```python
from build123d import *

# Parameters (mm, degrees)
SKETCH1_R           = 131
SKETCH1_R_2         = 126
BOSS_EXTRUDE1_DEPTH = 280
SKETCH4_R           = 140
SKETCH4_R_2         = 131
BOSS_EXTRUDE2_DEPTH = 9
CHAMFER1_SIZE       = 20
CHAMFER1_SIZE2      = 3.526539614
SKETCH5_R           = 132
SKETCH5_R_2         = 131
BOSS_EXTRUDE3_DEPTH = 15


with BuildPart() as part:
    # Sketch1 → Boss-Extrude1 (new body)
    with BuildSketch(Plane(origin=(0, 0, 0), x_dir=(1, 0, 0), z_dir=(0, 1, 0))):
        Circle(SKETCH1_R)
        Circle(SKETCH1_R_2, mode=Mode.SUBTRACT)
    extrude(amount=-BOSS_EXTRUDE1_DEPTH)

    # Sketch4 → Boss-Extrude2 (add)
    with BuildSketch(Plane(origin=(0, -12, 0), x_dir=(1, 0, 0), z_dir=(0, 1, 0))):
        Circle(SKETCH4_R)
        Circle(SKETCH4_R_2, mode=Mode.SUBTRACT)
    extrude(amount=-BOSS_EXTRUDE2_DEPTH)

    # Chamfer1
    chamfer1_edges = [part.edges().sort_by_distance(p)[0] for p in [
        (-126, -280, 0),
    ]]
    chamfer1_side = [part.faces().sort_by_distance(p)[0] for p in [
        (-126, -140, 0),
    ]]
    chamfer(chamfer1_edges, length=CHAMFER1_SIZE, length2=CHAMFER1_SIZE2, reference=chamfer1_side[0])

    # Sketch5 → Boss-Extrude3 (add)
    with BuildSketch(Plane.XZ.offset(21)):
        Circle(SKETCH5_R)
        Circle(SKETCH5_R_2, mode=Mode.SUBTRACT)
    extrude(amount=BOSS_EXTRUDE3_DEPTH)


solid = part.part
```
Can you work these out from the model? Positions are in its coordinate system, mm. A direction names the side the tool comes from. Round coordinates to 2 decimals unless told otherwise and drop trailing zeros. Loops run counter-clockwise (first coordinate to the right, second up) from the corner with the lowest first, then second, coordinate; pieces in that order, holes last.
Item 1: Will these pins go through, and if not, where does the flat tip stop? pin 1 Ø3 at (y, z) = (-245.5, 88.5) entering from +X; pin 2 Ø4 at (x, y) = (48, -43) entering from -Z; pin 3 Ø1 at (y, z) = (-193.5, 110.5) entering from +X.
Item 2: Suppose I cut it at C-C, the plane y = -87.5. Write out the boundary of the cut face in (x, z).
Item 3: Please list where these lines run through material, in increasing order: L1, parallel to Z at x = 0, y = -131; L2, parallel to X at y = -149.5, z = 17.
Item 4: If we mould it in two halves opening along Z, with no side actions, what happens to faces 1 (the cylindrical face through (121.934, -28.395, -50.557)), 2 (the conical face through (-27.36, -261.25, 123.22)), 3 (the flat face through (-127, -280, -30))? For each: +Z half, -Z half, draft (parallel to the pull), parting line (faces both ways), or undercut.
Item 5: Suppose I cut it at A-A, the plane x = 0. Write out the boundary of the cut face in (y, z), then the cut area to 3 significant figures.
Item 6: Suppose I cut it at B-B, the plane z = 0. Write out the boundary of the cut face in (x, y), then the cut area to 3 significant figures.
Item 7: Which directions (+Z, -Z, +X, -X, +Y, -Y) give clear straight access to the entire face, cutting with the end or side of a thin tool? Please do faces 4 (the cylindrical face through (124.95, -5.92, -39.35)), 5 (the flat face through (-69, 0, -107)), 6 (the flat face through (-94, -21, -94)).
Reported:
1. pin 1: stops at x = 97.94
1. pin 2: stops at z = -122.66
1. pin 3: stops at x = 71.14
2. outline: circle Ø262 at (0, 0); hole circle Ø252 at (0, 0)
3. L1: z = -131 to -126, 126 to 131
3. L2: x = -129.89 to -124.85, 124.85 to 129.89
4. face 1: parting line
4. face 2: undercut
4. face 3: draft
5. outline: (-280, -131) - (-36, -131) - (-36, -132) - (-21, -132) - (-21, -140) - (-12, -140) - (-12, -131) - (0, -131) - (0, -126) - (-260, -126) - (-280, -129.53) - close; (-280, 129.53) - (-260, 126) - (0, 126) - (0, 131) - (-12, 131) - (-12, 140) - (-21, 140) - (-21, 132) - (-36, 132) - (-36, 131) - (-280, 131) - close
5. area: 2,920 mm2
6. outline: (-140, -21) - (-132, -21) - (-132, -36) - (-131, -36) - (-131, -280) - (-129.53, -280) - (-126, -260) - (-126, 0) - (-131, 0) - (-131, -12) - (-140, -12) - close; (126, -260) - (129.53, -280) - (131, -280) - (131, -36) - (132, -36) - (132, -21) - (140, -21) - (140, -12) - (131, -12) - (131, 0) - (126, 0) - close
6. area: 2,920 mm2
7. face 4: +Y
7. face 5: +Z, -Z, +X, -X, +Y
7. face 6: -Y
